Source: CAD feature listing. Evaluate the final solid. Frame: model axes, mm. Face numbers are marked on the shaded views. A direction names the side the tool comes from. Give positions to 0.01 mm unless a question says otherwise; leave off trailing zeros. Order: outer loops, then holes, each group sorted by start corner. A loop starts at its lowest first (then second) coordinate and runs counter-clockwise, first axis right, second up. Notation, with made-up numbers: (50.5, 78.5) - (67.5, 78.5) arc R7 cw to (67.5, 83.5) - close; hole circle Ø10 at (-9.5, 37). An arc over 180 degrees is marked (long way). Answer as CSV lines item,"result".
```python
from build123d import *

# Parameters (mm, degrees)
F0_R     = 11
F1_DEPTH = 6


# Not quite as in the source:
# - a feature names something its author has since deleted; it is built from what else it names


with BuildPart() as f1:
    # F0 (on Top) → F1 (new body)
    with BuildSketch(Plane.XY):
        with BuildLine():
            ThreePointArc((1.8708277189, 36.7071093595), (1.9674419226, 36.3594054551), (2, 36))
            ThreePointArc((2, 36), (-0.3594054551, 34.0325580774), (-1.8708277189, 36.7071093595))
            Line((-1.8708277189, 36.7071093595), (-6.6345304801, 24.1035890545))
            ThreePointArc((-6.6345304801, 24.1035890545), (-14.1770019873, 8.1850959137), (-24.1915856836, -6.3061225893))
            Line((-24.1915856836, -6.3061225893), (-32.7247030643, -16.7333703491))
            ThreePointArc((-32.7247030643, -16.7333703491), (-30.5044478293, -16.116442587), (-29.1769145362, -18))
            ThreePointArc((-29.1769145362, -18), (-29.6527625783, -19.2949752156), (-30.8538753454, -19.9737390104))
            Line((-30.8538753454, -19.9737390104), (-17.5570552035, -17.7974664652))
            ThreePointArc((-17.5570552035, -17.7974664652), (0, -16.3701918273), (17.5570552035, -17.7974664652))
            Line((17.5570552035, -17.7974664652), (30.8538753454, -19.9737390104))
            ThreePointArc((30.8538753454, -19.9737390104), (29.4448637287, -17), (32.7247030643, -16.7333703491))
            Line((32.7247030643, -16.7333703491), (24.1915856836, -6.3061225893))
            ThreePointArc((24.1915856836, -6.3061225893), (14.1770019873, 8.1850959137), (6.6345304801, 24.1035890545))
            Line((6.6345304801, 24.1035890545), (1.8708277189, 36.7071093595))
        make_face()
        with BuildLine():
            ThreePointArc((-18.4064805015, -14.9474780208), (-20.765299785, -14.6147639762), (-22.5166604984, -13))
            Line((-22.5166604984, -13), (-12.3317924474, -7.1197636891))
            ThreePointArc((-12.3317924474, -7.1197636891), (-9.7788523145, -10.4437050957), (-6.4502961482, -12.9906255195))
            Line((-6.4502961482, -12.9906255195), (-18.4064805015, -14.9474780208))
        make_face(mode=Mode.SUBTRACT)
        with BuildLine():
            ThreePointArc((22.1481359393, -8.4667406982), (23.0394067662, -10.6758951429), (22.5166604984, -13))
            Line((22.5166604984, -13), (12.3317924474, -7.1197636891))
            ThreePointArc((12.3317924474, -7.1197636891), (13.9339400798, -3.2468819763), (14.4753597851, 0.9091924335))
            Line((14.4753597851, 0.9091924335), (22.1481359393, -8.4667406982))
        make_face(mode=Mode.SUBTRACT)
        Circle(F0_R, mode=Mode.SUBTRACT)
        with BuildLine():
            ThreePointArc((-3.7416554378, 23.414218719), (-2.2741069812, 25.2906591191), (0, 26))
            Line((0, 26), (0, 14.2395273782))
            ThreePointArc((0, 14.2395273782), (-4.1550877653, 13.6905870721), (-8.0250636368, 12.0814330861))
            Line((-8.0250636368, 12.0814330861), (-3.7416554378, 23.414218719))
        make_face(mode=Mode.SUBTRACT)
        with BuildLine():
            ThreePointArc((-1.8708277189, 36.7071093595), (-0.3594054551, 34.0325580774), (2, 36))
            ThreePointArc((2, 36), (1.9674419226, 36.3594054551), (1.8708277189, 36.7071093595))
            ThreePointArc((1.8708277189, 36.7071093595), (0, 38), (-1.8708277189, 36.7071093595))
        make_face()
        with BuildLine():
            ThreePointArc((33.1769145362, -18), (33.0604719492, -17.327533293), (32.7247030643, -16.7333703491))
            ThreePointArc((32.7247030643, -16.7333703491), (29.4448637287, -17), (30.8538753454, -19.9737390104))
            ThreePointArc((30.8538753454, -19.9737390104), (32.4718897519, -19.5241519579), (33.1769145362, -18))
        make_face()
        with BuildLine():
            ThreePointArc((-29.1769145362, -18), (-30.5044478293, -16.116442587), (-32.7247030643, -16.7333703491))
            ThreePointArc((-32.7247030643, -16.7333703491), (-32.9089653438, -19), (-30.8538753454, -19.9737390104))
            ThreePointArc((-30.8538753454, -19.9737390104), (-29.6527625783, -19.2949752156), (-29.1769145362, -18))
        make_face()
    extrude(amount=F1_DEPTH)


solid = f1.part
```
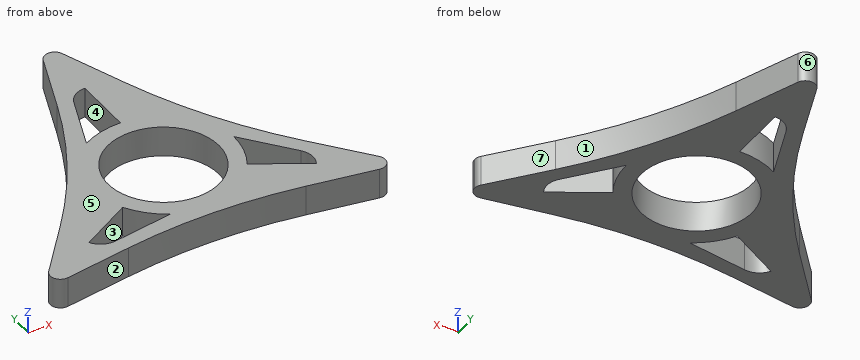
(1) Cut plane A-A (z = 3). Return loops of the section in (x, y), then the cut area to 3 significant figures.
Completed:
outline,"(-32.72, -16.73) arc R2 ccw to (-30.85, -19.97) - (-17.56, -17.8) arc R108.7 cw to (17.56, -17.8) - (30.85, -19.97) arc R2 ccw to (32.72, -16.73) - (24.19, -6.31) arc R108.7 cw to (6.63, 24.1) - (1.87, 36.71) arc R2 ccw to (-1.87, 36.71) - (-6.63, 24.1) arc R108.7 cw to (-24.19, -6.31) - close; hole (-22.52, -13) arc R4 ccw to (-18.41, -14.95) - (-6.45, -12.99) arc R16 cw to (-12.33, -7.12) - close; hole circle Ø22 at (0, 0); hole (-8.03, 12.08) arc R16 cw to (0, 14.24) - (0, 26) arc R4 ccw to (-3.74, 23.41) - close; hole (12.33, -7.12) - (22.52, -13) arc R4 ccw to (22.15, -8.47) - (14.48, 0.91) arc R16 cw to start"
area,"1,080 mm²"
(2) Access query for the marked faces 1, 2 and 3. Directions: +Z, -Z, +X, -X, +Y, -Y. A direction counts if a zero-diameter tool reaches every point of the face in a straight line with its end or side. Return the directions, or none.
Completed:
face 1,"+Z, -Z, +X, +Y"
face 2,"+Z, -Z, -Y"
face 3,"+Z, -Z"
(3) Cut plane D-D (x = 4). Return loops of the section in (y, z), then the cut area to 3 significant figures.
Completed:
outline,"(-16.44, 0) - (-10.25, 0) - (-10.25, 6) - (-16.44, 6) - close; (10.25, 0) - (31.07, 0) - (31.07, 6) - (10.25, 6) - close"
area,"162 mm²"
(4) Contact query for flat-ended pins moving along their axis: pin 1 (10 mm diameter, centred on x = 9.5, y = 25, fed in from -Z); pin 2 (17.5 mm diameter, centred on x = 0, y = 0, fed in from +Z); pin 3 (1.5 mm diameter, centred on x = 2.5, z = 5.5, fed in from +Y); pin 4 (1.5 mm diameter, centred on y = 26, z = 2, fed in from -X). Output: stop coordinate, or through.
Completed:
pin 1,"z = 0"
pin 2,"through"
pin 3,"y = 36.97"
pin 4,"x = -6.2"
(5) Mould query, pull axis X, two halves, no side actions, for the marked faces 4, 5, 6 and 7. Classes: released by +X, released by -X, zero draft, split by the parting line, or undercut.
Completed:
face 4,"undercut"
face 5,"zero draft"
face 6,"split by the parting line"
face 7,"released by +X"
(6) Ray query, line 1 (Y direction, x = -1.5, z = 4); line 2 (Y direction, x = 20, z = 5.5); line 3 (Y direction, x = 15, z = 5.15). Return the intervals inside material, ascending. Write a range as from..to.
Completed:
line 1,"-16.38..-10.9, 10.9..14.17, 25.71..37.32"
line 2,"-18.2..-11.55, -5.84..-0.84"
line 3,"-17.41..-8.66, 0.27..6.78"
(7) Cut plane B-B (y = 21). Return loops of the section in (x, z).
Completed:
outline,"(-7.86, 0) - (-4.65, 0) - (-4.65, 6) - (-7.86, 6) - close; (0, 0) - (7.86, 0) - (7.86, 6) - (0, 6) - close"
(8) Cut plane C-C (y = -12). Return loops of the section in (x, z).
Completed:
outline,"(-28.85, 0) - (-20.78, 0) - (-20.78, 6) - (-28.85, 6) - close; (-7.97, 0) - (20.78, 0) - (20.78, 6) - (-7.97, 6) - close; (22.93, 0) - (28.85, 0) - (28.85, 6) - (22.93, 6) - close"
